Check sheet for the drawn part. Datum: minimum x, y, z corner. Units: mm. Coordinates: 2 decimals unless noted, no trailing zeros. Loops run counter-clockwise (first coordinate to the right, second up) from the corner with the lowest first, then second, coordinate; pieces in that order, holes last.
Q1. Sectioned sample at D-D (y = 10). Enter the section's corners in (x, z), then the cut area to 3 significant figures.
Q2. Sectioned sample at C-C (y = 6). Enter the section's corners in (x, z), then the cut area to 3 significant figures.
Q3. Sectioned sample at A-A (x = 10). Enter the section's corners in (y, z).
Q4. Go/stop test with a flat-tipped pin: P1, Ø1, axis at y = 9.5, z = 2, coming from the -X side. Record where the tip stops, or that it passes through.
Q5. Mould release check, pull along X, two halves, no side actions. Record for the marked faces 1, 2, 3 and 4: +X half, -X half, draft (parallel to the pull), parting line (faces both ways), or undercut.
Q6. Sectioned sample at B-B (z = 2.9). Enter the section's corners in (x, y), then the cut area to 3 significant figures.
Q7. Material ranges on probe 1 along Y at (x, z) = (10, 1.5); probe 2 along X at (y, z) = (11.5, 0.6); probe 3 along Y at (x, z) = (37.5, 3.1), recorded low to high.
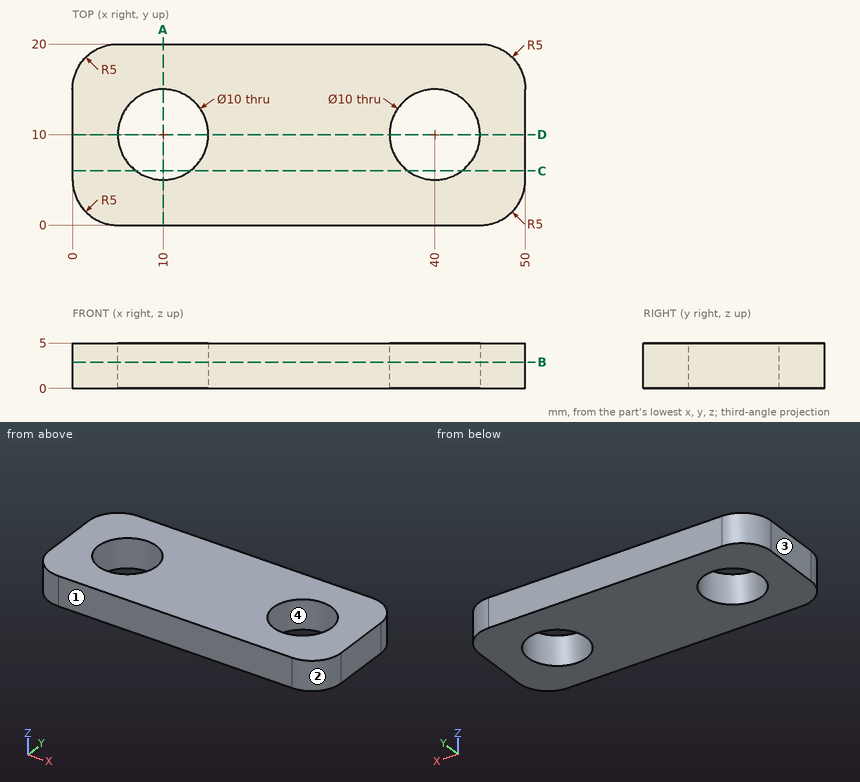
Geometry check:
1. outline: (0, 0) - (5, 0) - (5, 5) - (0, 5) - close; (15, 0) - (35, 0) - (35, 5) - (15, 5) - close; (45, 0) - (50, 0) - (50, 5) - (45, 5) - close
1. area: 150 mm2
2. outline: (0, 0) - (7, 0) - (7, 5) - (0, 5) - close; (13, 0) - (37, 0) - (37, 5) - (13, 5) - close; (43, 0) - (50, 0) - (50, 5) - (43, 5) - close
2. area: 190 mm2
3. outline: (0, 0) - (5, 0) - (5, 5) - (0, 5) - close; (15, 0) - (20, 0) - (20, 5) - (15, 5) - close
4. P1: stops at x = 0
5. face 1: draft
5. face 2: +X half
5. face 3: -X half
5. face 4: undercut
6. outline: (0, 5) arc R5 ccw to (5, 0) - (45, 0) arc R5 ccw to (50, 5) - (50, 15) arc R5 ccw to (45, 20) - (5, 20) arc R5 ccw to (0, 15) - close; hole circle Ø10 at (10, 10); hole circle Ø10 at (40, 10)
6. area: 821 mm2
7. probe 1: y = 0 to 5, 15 to 20
7. probe 2: x = 0 to 5.23, 14.77 to 35.23, 44.77 to 50
7. probe 3: y = 0 to 5.67, 14.33 to 20
